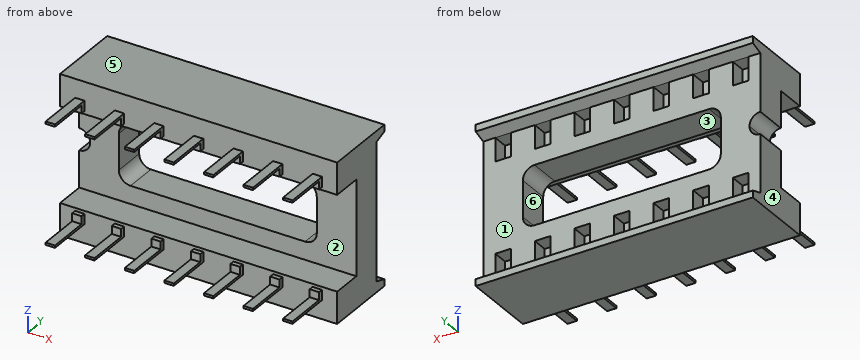
from build123d import *

# Parameters (mm, degrees)
EXTRUDE_1_DEPTH     = 8.89
CUT_EXTRUDE_1_REACH = 14.417
CUT_EXTRUDE_2_REACH = 14.417
SKETCH_3_4_W        = 1
SKETCH_3_4_H        = 1.5
CUT_EXTRUDE_3_DEPTH = 1
SKETCH_4_W          = 0.97
SKETCH_4_H          = 3
SKETCH_4_W_2        = 1.94
CUT_EXTRUDE_4_DEPTH = 14.507158287


with BuildPart() as part:
    # Эскиз2 → Бобышка-Вытянуть1 (new, symmetric)
    with BuildSketch(Plane(origin=(0, 0, 0), x_dir=(0, 0, -1), z_dir=(1, 0, 0))):
        Polygon((4.399571873, 4.024999392), (-4.399571873, 4.024999392), (-4.64484088, 4.8), (-5.08, 4.8), (-5.08, 0), (-3.885, 0), (-3.885, -3), (-3.735, -3), (-3.735, -0.3), (-3.235, -0.3), (-3.235, 0), (-3.045579843, 0), (-3.045579843, 1.95423056), (3.045579843, 1.95423056), (3.045579843, 0), (3.235, 0), (3.235, -0.3), (3.735, -0.3), (3.735, -3), (3.885, -3), (3.885, 0), (5.08, 0), (5.08, 4.8), (4.64484088, 4.8), align=None)
    extrude(amount=EXTRUDE_1_DEPTH, both=True)

    # Эскиз3 → Вырез-Вытянуть1 (cut, up to next)
    with BuildSketch(Plane(origin=(0, 4.024999392, 0), x_dir=(1, 0, 0), z_dir=(0, 1, 0)), mode=Mode.PRIVATE) as cut_extrude_1_sk1:
        with BuildLine():
            Line((-8.89, 0.7), (-8.89, 0))
            Line((-8.89, 0), (-8.19, 0))
            ThreePointArc((-8.19, 0), (-8.395025253, 0.494974747), (-8.89, 0.7))
        make_face()
    cut_extrude_1_tool1 = extrude(cut_extrude_1_sk1.sketch, amount=-CUT_EXTRUDE_1_REACH, mode=Mode.PRIVATE) & part.part
    # Эскиз3 → Вырез-Вытянуть1 (cut, up to next)
    with BuildSketch(Plane(origin=(0, 4.024999392, 0), x_dir=(1, 0, 0), z_dir=(0, 1, 0)), mode=Mode.PRIVATE) as cut_extrude_1_sk2:
        with BuildLine():
            Line((-8.19, 0), (-8.89, 0))
            Line((-8.89, 0), (-8.89, -0.7))
            ThreePointArc((-8.89, -0.7), (-8.395025253, -0.494974747), (-8.19, 0))
        make_face()
    cut_extrude_1_tool2 = extrude(cut_extrude_1_sk2.sketch, amount=-CUT_EXTRUDE_1_REACH, mode=Mode.PRIVATE) & part.part
    # Эскиз3 → Вырез-Вытянуть1 (cut, up to next)
    with BuildSketch(Plane(origin=(0, 4.024999392, 0), x_dir=(1, 0, 0), z_dir=(0, 1, 0)), mode=Mode.PRIVATE) as cut_extrude_1_sk3:
        with BuildLine():
            Line((-8.89, 0.7), (-8.89, 0))
            Line((-8.89, 0), (-8.19, 0))
            ThreePointArc((-8.19, 0), (-8.395025253, 0.494974747), (-8.89, 0.7))
        make_face()
    cut_extrude_1_tool3 = extrude(cut_extrude_1_sk3.sketch, amount=-CUT_EXTRUDE_1_REACH, mode=Mode.PRIVATE) & part.part
    # Эскиз3 → Вырез-Вытянуть1 (cut, up to next)
    with BuildSketch(Plane(origin=(0, 4.024999392, 0), x_dir=(1, 0, 0), z_dir=(0, 1, 0)), mode=Mode.PRIVATE) as cut_extrude_1_sk4:
        with BuildLine():
            Line((-8.19, 0), (-8.89, 0))
            Line((-8.89, 0), (-8.89, -0.7))
            ThreePointArc((-8.89, -0.7), (-8.395025253, -0.494974747), (-8.19, 0))
        make_face()
    cut_extrude_1_tool4 = extrude(cut_extrude_1_sk4.sketch, amount=-CUT_EXTRUDE_1_REACH, mode=Mode.PRIVATE) & part.part
    add(cut_extrude_1_tool1.solids().sort_by_distance((-8.592911, 4.024999, -0.297089))[0], mode=Mode.SUBTRACT)
    add(cut_extrude_1_tool2.solids().sort_by_distance((-8.592911, 4.024999, 0.297089))[0], mode=Mode.SUBTRACT)
    add(cut_extrude_1_tool3.solids().sort_by_distance((-8.592911, 4.024999, -0.297089))[0], mode=Mode.SUBTRACT)
    add(cut_extrude_1_tool4.solids().sort_by_distance((-8.592911, 4.024999, 0.297089))[0], mode=Mode.SUBTRACT)

    # Эскиз3<3> → Вырез-Вытянуть2 (cut, up to next)
    with BuildSketch(Plane(origin=(0, 4.024999392, 0), x_dir=(1, 0, 0), z_dir=(0, 1, 0)), mode=Mode.PRIVATE) as cut_extrude_2_sk1:
        with BuildLine():
            Line((6.35, 0), (-6.35, 0))
            Line((-6.35, 0), (-6.35, -1.149571873))
            ThreePointArc((-6.35, -1.149571873), (-6.130330086, -1.679901959), (-5.6, -1.899571873))
            Line((-5.6, -1.899571873), (5.6, -1.899571873))
            ThreePointArc((5.6, -1.899571873), (6.130330086, -1.679901959), (6.35, -1.149571873))
            Line((6.35, -1.149571873), (6.35, 0))
        make_face()
    cut_extrude_2_tool1 = extrude(cut_extrude_2_sk1.sketch, amount=-CUT_EXTRUDE_2_REACH, mode=Mode.PRIVATE) & part.part
    # Эскиз3<3> → Вырез-Вытянуть2 (cut, up to next)
    with BuildSketch(Plane(origin=(0, 4.024999392, 0), x_dir=(1, 0, 0), z_dir=(0, 1, 0)), mode=Mode.PRIVATE) as cut_extrude_2_sk2:
        with BuildLine():
            Line((-6.35, 1.149571873), (-6.35, 0))
            Line((-6.35, 0), (6.35, 0))
            Line((6.35, 0), (6.35, 1.149571873))
            ThreePointArc((6.35, 1.149571873), (6.130330086, 1.679901959), (5.6, 1.899571873))
            Line((5.6, 1.899571873), (-5.6, 1.899571873))
            ThreePointArc((-5.6, 1.899571873), (-6.130330086, 1.679901959), (-6.35, 1.149571873))
        make_face()
    cut_extrude_2_tool2 = extrude(cut_extrude_2_sk2.sketch, amount=-CUT_EXTRUDE_2_REACH, mode=Mode.PRIVATE) & part.part
    add(cut_extrude_2_tool1.solids().sort_by_distance((0, 4.024999, 0.941878))[0], mode=Mode.SUBTRACT)
    add(cut_extrude_2_tool2.solids().sort_by_distance((0, 4.024999, -0.941878))[0], mode=Mode.SUBTRACT)

    # Эскиз3<4> → Вырез-Вытянуть3 (cut)
    with BuildSketch(Plane(origin=(0, 4.024999392, 0), x_dir=(1, 0, 0), z_dir=(0, 1, 0))):
        with Locations((-7.62, 3.649571873)):
            Rectangle(SKETCH_3_4_W, SKETCH_3_4_H)
        with Locations((-5.08, 3.649571873)):
            Rectangle(SKETCH_3_4_W, SKETCH_3_4_H)
        with Locations((-2.54, 3.649571873)):
            Rectangle(SKETCH_3_4_W, SKETCH_3_4_H)
        with Locations((0, 3.649571873)):
            Rectangle(SKETCH_3_4_W, SKETCH_3_4_H)
        with Locations((2.54, 3.649571873)):
            Rectangle(SKETCH_3_4_W, SKETCH_3_4_H)
        with Locations((5.08, 3.649571873)):
            Rectangle(SKETCH_3_4_W, SKETCH_3_4_H)
        with Locations((7.62, 3.649571873)):
            Rectangle(SKETCH_3_4_W, SKETCH_3_4_H)
        with Locations((7.62, -3.649571873)):
            Rectangle(SKETCH_3_4_W, SKETCH_3_4_H)
        with Locations((5.08, -3.649571873)):
            Rectangle(SKETCH_3_4_W, SKETCH_3_4_H)
        with Locations((2.54, -3.649571873)):
            Rectangle(SKETCH_3_4_W, SKETCH_3_4_H)
        with Locations((0, -3.649571873)):
            Rectangle(SKETCH_3_4_W, SKETCH_3_4_H)
        with Locations((-2.54, -3.649571873)):
            Rectangle(SKETCH_3_4_W, SKETCH_3_4_H)
        with Locations((-5.08, -3.649571873)):
            Rectangle(SKETCH_3_4_W, SKETCH_3_4_H)
        with Locations((-7.62, -3.649571873)):
            Rectangle(SKETCH_3_4_W, SKETCH_3_4_H)
    extrude(amount=-CUT_EXTRUDE_3_DEPTH, mode=Mode.SUBTRACT)

    # Эскиз4 → Вырез-Вытянуть4 (cut, through all)
    with BuildSketch(Plane.XY.offset(3.885)):
        with Locations((-8.405, -1.5)):
            Rectangle(SKETCH_4_W, SKETCH_4_H)
        with Locations((-6.35, -1.5)):
            Rectangle(SKETCH_4_W_2, SKETCH_4_H)
        with Locations((-3.81, -1.5)):
            Rectangle(SKETCH_4_W_2, SKETCH_4_H)
        with Locations((-1.27, -1.5)):
            Rectangle(SKETCH_4_W_2, SKETCH_4_H)
        with Locations((1.27, -1.5)):
            Rectangle(SKETCH_4_W_2, SKETCH_4_H)
        with Locations((3.81, -1.5)):
            Rectangle(SKETCH_4_W_2, SKETCH_4_H)
        with Locations((6.35, -1.5)):
            Rectangle(SKETCH_4_W_2, SKETCH_4_H)
        with Locations((8.405, -1.5)):
            Rectangle(SKETCH_4_W, SKETCH_4_H)
    extrude(amount=-CUT_EXTRUDE_4_DEPTH, mode=Mode.SUBTRACT)


solid = part.part
Read the model definition and answer for the solid it produces. Units are mm, in the model's axes. Face numbers are marked on the shaded views. A direction names the side the tool comes from. Round coordinates to 2 decimals unless told otherwise and drop trailing zeros. Loops run counter-clockwise (first coordinate to the right, second up) from the corner with the lowest first, then second, coordinate; pieces in that order, holes last. Notation, with made-up numbers: (9, 21) - (33, 21) arc R28 ccw to (33, 52) - close; hole circle Ø2 at (10.25, -13.75). An arc over 180 degrees is marked (long way). One line per question, with ' | ' between items. Start each with the question number.
Q1. For the marked faces 1, 2 and 3, determine the directions among +Z, -Z, +X, -X, +Y, -Y from which every point of the face is accessible in a straight line to the end or side of a thin tool.
Q2. Flat-ended cylindrical pins translate along their axes: pin 1 (0.5 mm diameter, centred on x = -2.5, y = -1, fed in from +Z) (3 decimals); pin 2 (0.7 mm diameter, centred on y = -2, z = -3.5, fed in from -X). Find the tip coordinate at first contact, or state that the pin passes through.
Q3. Section C-C on z = -0.5 is taken. Give the vertices of the cut face in (x, y) (3 decimals), plus the area to 3 significant figures.
Q4. Find the intervals of material crossed by L1, parallel to Z at x = 7.75, y = 0.5; L2, parallel to Z at x = -3.75, y = 3; L3, parallel to X at y = 3, z = -1, in increasing order.
Q5. Section B-B on x = -3.25 is taken. Give the vertices of the cut face in (y, z) (3 decimals), plus the area to 3 significant figures.
Q6. For a pull along X with two mould halves and no side action, classify the marked faces 4, 5 and 6 as +X half, -X half, draft (parallel to the pull), parting line (faces both ways), or undercut.
Q7. Section A-A on y = 0.5 is taken. Give the vertices of the cut face in (x, z).
Q8. Section D-D on y = 2.5 is taken. Give the vertices of the cut face in (x, z).
Established:
1) face 1: +X, -X, +Y | face 2: +X, -X, -Y | face 3: +Y, -Y
2) pin 1: z = 3.885 | pin 2: x = -7.92
3) outline: (-8.4, 1.954) - (-6.35, 1.954) - (-6.35, 4.025) - (-8.4, 4.025) - close; (6.35, 1.954) - (8.89, 1.954) - (8.89, 4.025) - (6.35, 4.025) - close | area: 9.51 mm²
4) L1: -5.08 to -3.05, 3.05 to 5.08 | L2: -5.08 to -1.9, 1.9 to 5.08 | L3: -8.89 to -6.35, 6.35 to 8.89
5) outline: (0, -5.08) - (4.8, -5.08) - (4.8, -4.645) - (4.025, -4.4) - (4.025, -1.9) - (1.954, -1.9) - (1.954, -3.046) - (0, -3.046) - close; (0, 3.046) - (1.954, 3.046) - (1.954, 1.9) - (4.025, 1.9) - (4.025, 4.4) - (4.8, 4.645) - (4.8, 5.08) - (0, 5.08) - close | area: 22.0 mm²
6) face 4: -X half | face 5: draft | face 6: undercut
7) outline: (-8.89, -5.08) - (8.89, -5.08) - (8.89, -3.05) - (-8.89, -3.05) - close; (-8.89, 3.05) - (8.89, 3.05) - (8.89, 5.08) - (-8.89, 5.08) - close
8) outline: (-8.89, -5.08) - (8.89, -5.08) - (8.89, 5.08) - (-8.89, 5.08) - (-8.89, 0.7) arc R0.7 cw to (-8.89, -0.7) - close; hole (-6.35, -1.15) arc R0.75 ccw to (-5.6, -1.9) - (5.6, -1.9) arc R0.75 ccw to (6.35, -1.15) - (6.35, 1.15) arc R0.75 ccw to (5.6, 1.9) - (-5.6, 1.9) arc R0.75 ccw to (-6.35, 1.15) - close
